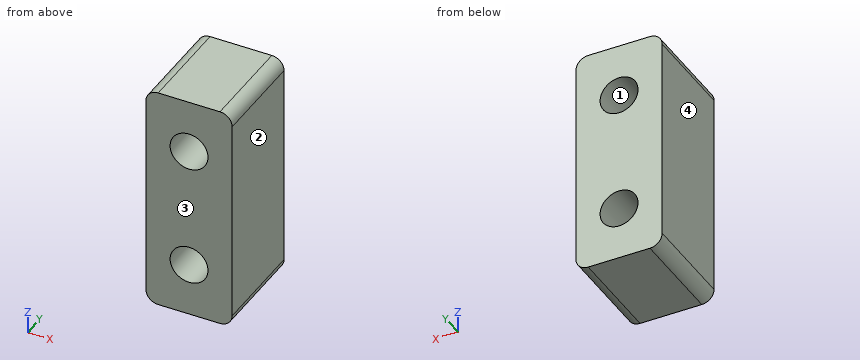
Autodesk Inventor part; units mm, degrees
ref_plane "YZ Plane" through (0, 0, 0) normal (1, 0, 0) x (0, 1, 0)
ref_plane "XZ Plane" through (0, 0, 0) normal (0, 1, 0) x (-1, 0, 0)
ref_plane "XY Plane" through (0, 0, 0) normal (0, 0, 1) x (1, 0, 0)
sketch "Эскиз1" plane through (0, 0, 0) normal (0, 1, 0) x (-1, 0, 0)
  circle A0 centre (0, -5) radius 1.55
  circle A1 centre (0, 5) radius 1.55
  line L0 (0, 5) -> (0, -5) construction
  line L1 (3.525, 9.35) -> (-3.525, 9.35)
  line L2 (-3.525, 9.35) -> (-3.525, -9.35)
  line L3 (-3.525, -9.35) -> (3.525, -9.35)
  line L4 (3.525, -9.35) -> (3.525, 9.35)
  line L5 (3.525, 9.35) -> (-3.525, -9.35) construction
  line L6 (-3.525, 9.35) -> (3.525, -9.35) construction
  point P0 (0, 0)
  point P1 (0, 0)
  dimension "d2" = 3.1
  dimension "d3" = 3.1
  dimension "d4" = 10
  dimension "d5" = 7.05
  dimension "d6" = 18.7
extrude "Выдавливание1" add sketch "Эскиз1" along normal blind 8
fillet "Сопряжение1" radius 1 4 edges at (-3.525, 4, 9.35) (3.525, 4, 9.35) (3.525, 4, -9.35) (-3.525, 4, -9.35)
properties part number "креп_сервы"
Work out the finished part from the listing and answer in its coordinate system (mm). Face numbers are marked on the shaded views. Coordinates: 2 decimals unless noted, no trailing zeros. Write each loop counter-clockwise with the first axis right and the second up, starting at its lowest first coordinate (ties: lowest second). Pieces come first, ordered by that corner, then holes. Notation, with made-up numbers: (-32.5, 86.5) - (19.5, 86.5) arc R12 cw to (19.5, 94.5) - close; hole circle Ø9 at (6.5, 22.25). An arc over 180 degrees is marked (long way). One line per question, with ' | ' between items.
1) Find section A-A, the plane x = 0. Determine the outline of the cut face in (y, z).
Checks:
outline: (0, -9.35) - (8, -9.35) - (8, -6.55) - (0, -6.55) - close; (0, -3.45) - (8, -3.45) - (8, 3.45) - (0, 3.45) - close; (0, 6.55) - (8, 6.55) - (8, 9.35) - (0, 9.35) - close
2) Find section B-B, the plane z = 5. Determine the outline of the cut face in (x, y) (3 decimals).
Checks:
outline: (-3.525, 0) - (-1.55, 0) - (-1.55, 8) - (-3.525, 8) - close; (1.55, 0) - (3.525, 0) - (3.525, 8) - (1.55, 8) - close
3) Find section C-C, the plane y = 4. Determine the outline of the cut face in (x, z) (3 decimals), and give its area (3 significant figures).
Checks:
outline: (-3.525, -8.35) arc R1 ccw to (-2.525, -9.35) - (2.525, -9.35) arc R1 ccw to (3.525, -8.35) - (3.525, 8.35) arc R1 ccw to (2.525, 9.35) - (-2.525, 9.35) arc R1 ccw to (-3.525, 8.35) - close; hole circle Ø3.1 at (0, -5); hole circle Ø3.1 at (0, 5) | area: 116 mm2
4) Consider probe 1 along Z at (x, y) = (0, 4.5); probe 2 along Z at (x, y) = (-1, 5.75); probe 3 along X at (y, z) = (7.5, 5.75) (3 decimals). Determine where each line is inside the solid, lowest interval first. Write a range as [from, to].
Checks:
probe 1: [-9.35, -6.55], [-3.45, 3.45], [6.55, 9.35] | probe 2: [-9.35, -6.18], [-3.82, 3.82], [6.18, 9.35] | probe 3: [-3.525, -1.356], [1.356, 3.525]
5) Find section D-D, the plane x = 1. Determine the outline of the cut face in (y, z), and give its area (3 significant figures).
Checks:
outline: (0, -9.35) - (8, -9.35) - (8, -6.18) - (0, -6.18) - close; (0, -3.82) - (8, -3.82) - (8, 3.82) - (0, 3.82) - close; (0, 6.18) - (8, 6.18) - (8, 9.35) - (0, 9.35) - close | area: 112 mm2
6) The mould has two halves that part along X. Classify the marked faces 1, 2, 3 and 4: +X half, -X half, draft (parallel to the pull), parting line (faces both ways), or undercut.
Checks:
face 1: undercut | face 2: +X half | face 3: draft | face 4: -X half
